```python
from build123d import *

# Parameters (mm, degrees)
ESBO_O3_R                = 2.5
RESSALTO_EXTRUS_O1_DEPTH = 7.89
ESBO_O4_W                = 8
ESBO_O4_H                = 12
RESSALTO_EXTRUS_O2_DEPTH = 10
FILETE1_R                = 10
VARREDURA1_START         = -2.055
VARREDURA1_DEPTH         = 4.5
FILETE2_R                = 10
FILETE3_R                = 1
FILETE2_OF_ESPELHAR1_R   = 10
FILETE3_OF_ESPELHAR1_R   = 1


# Read off the part's stored shape, not the designer's step: Varredura1
with BuildPart() as part:
    # Esboço3 → Ressalto-extrusão1 (new body)
    with BuildSketch(Plane.XY):
        with BuildLine():
            Line((-4, 0), (-4, 12))
            Line((-4, 12), (4, 12))
            Line((4, 12), (4, 0))
            ThreePointArc((4, 0), (0, -4), (-4, 0))
        make_face()
        Circle(ESBO_O3_R, mode=Mode.SUBTRACT)
    extrude(amount=RESSALTO_EXTRUS_O1_DEPTH)

    # Esboço4 → Ressalto-extrusão2 (add)
    with BuildSketch(Plane(origin=(0, 12, 0), x_dir=(1, 0, 0), z_dir=(0, 1, 0))):
        with Locations((0, -3.945)):
            Rectangle(ESBO_O4_W, ESBO_O4_H)
    extrude(amount=RESSALTO_EXTRUS_O2_DEPTH)

    # Filete1
    # the kernel refuses this fillet: 10 mm, written as the material it adds along each edge
    with BuildSketch(Plane(origin=(-4, 12, 0), x_dir=(0, 0, -1), z_dir=(1, 0, 0))) as filete1_piece_1:
        with BuildLine():
            CenterArc((10, -6.072641517), FILETE1_R, 142.608054869, 37.391945131)
            Line((0, -6.072641517), (-0.2, -6.072641517))
            Line((-0.2, -6.072641517), (-0.2, 0))
            Line((-0.2, 0), (0, 0.2))
            ThreePointArc((0, 0.2), (1.0275, 0.2), (1.8961, 0.12145283))
            Line((1.8961, 0.12145283), (2.055, 0))
        make_face()
    extrude(amount=8)
    with BuildSketch(Plane(origin=(-4, 12, 7.89), x_dir=(0, 0, 1), z_dir=(1, 0, 0))) as filete1_piece_2:
        with BuildLine():
            CenterArc((10, 6.072641517), FILETE1_R, 180, 37.391945131)
            Line((0, 6.072641517), (-0.2, 6.072641517))
            Line((-0.2, 6.072641517), (-0.2, 0))
            Line((-0.2, 0), (0, -0.2))
            ThreePointArc((0, -0.2), (1.0275, -0.2), (1.8961, -0.12145283))
            Line((1.8961, -0.12145283), (2.055, 0))
        make_face()
    extrude(amount=8)

    # Varredura1 outline → Varredura1 (add)
    with BuildSketch(Plane.XY.offset(VARREDURA1_START)):
        with BuildLine():
            Line((-4, 22), (4, 22))
            add(Edge.make_bspline(
                [(4, 22), (4.076004643, 24.789100523), (4.576744422, 27.046075873), (5.825537248, 29.832679333), (6.324748717, 30.661737223), (7.465829447, 32.153454516), (8.107698711, 32.816113914), (10.212438301, 34.604326425), (11.854440436, 35.53011384), (15.430236778, 37.114751087), (17.364030989, 37.773600914), (19.350774872, 38.4318674)],
                knots=[0, 0, 0, 0, 0.25, 0.25, 0.375, 0.375, 0.5, 0.5, 0.75, 0.75, 1, 1, 1, 1], degree=3))
            Line((19.350774872, 38.4318674), (16.628722538, 45.954528571))
            add(Edge.make_bspline(
                [(-4, 22), (-3.924365702, 25.610706729), (-3.278889097, 28.990240165), (-1.326924275, 33.467921051), (-0.516042652, 34.853906552), (1.338266133, 37.332612564), (2.378280036, 38.423434753), (5.639368368, 41.249638523), (7.969155498, 42.540719328), (12.436975606, 44.550100168), (14.600059443, 45.281114301), (16.628722538, 45.954528571)],
                knots=[0, 0, 0, 0, 0.25, 0.25, 0.375, 0.375, 0.5, 0.5, 0.75, 0.75, 1, 1, 1, 1], degree=3))
        make_face()
    varredura1 = extrude(amount=VARREDURA1_DEPTH)

    # Filete2
    # the kernel refuses this fillet: 10 mm, written as the material it takes off along each edge
    with BuildSketch(Plane(origin=(19.350774872, 38.4318674, -22.846513703), x_dir=(-0.9279643931477312, -0.3726688678303612, 8.125821655605385e-13), z_dir=(0, 2.1804401593599865e-12, 1.0))) as filete2_piece_1:
        with BuildLine():
            CenterArc((9.534418095, -9.925569628), FILETE2_R, 96.994915397, 71.874930906)
            Line((-0.277493979, -7.99518587), (-0.473732221, -7.956578195))
            ThreePointArc((-0.473732221, -7.956578195), (-0.338626636, -3.990655585), (-0.199879647, 0.006937349))
            Line((-0.199879647, 0.006937349), (0.012379593, 0.199616497))
            ThreePointArc((0.012379593, 0.199616497), (4.158510673, 0.013875219), (8.292249229, 0.198511393))
            Line((8.292249229, 0.198511393), (8.316605481, 0))
        make_face()
    extrude(amount=46.083027405, mode=Mode.SUBTRACT)

    # Filete3
    filete3_edges = [part.edges().sort_by_distance(p)[0] for p in [
        (16.628722538, 45.954528571, 0.195),
    ]]
    fillet(filete3_edges, radius=FILETE3_R)

    # Espelhar1: Varredura1 across plane
    add(varredura1.mirror(Plane.XY.offset(4)))

    # Filete2 of Espelhar1
    # the kernel refuses this fillet: 10 mm, written as the material it takes off along each edge
    with BuildSketch(Plane(origin=(19.350774872, 38.4318674, 30.846513703), x_dir=(-0.34025654174280723, 0.9403326463551213, 2.0503390652699583e-12), z_dir=(0, 2.1804401593599865e-12, -1.0))) as filete2_of_espelhar1_piece_1:
        with BuildLine():
            CenterArc((9.588878802, -9.87296633), FILETE2_OF_ESPELHAR1_R, 99.142350717, 71.874930906)
            Line((-0.288475994, -8.311600828), (-0.48602309, -8.280373518))
            ThreePointArc((-0.48602309, -8.280373518), (-0.158112079, -4.155526935), (-0.199925782, -0.005448096))
            Line((-0.199925782, -0.005448096), (0, 0.2))
            ThreePointArc((0, 0.2), (4, 0.2), (7.968222424, 0.197459327))
            Line((7.968222424, 0.197459327), (8, 0))
        make_face()
    extrude(amount=46.083027405, mode=Mode.SUBTRACT)

    # Filete3 of Espelhar1
    filete3_of_espelhar1_edges = [part.edges().sort_by_distance(p)[0] for p in [
        (16.628722538, 45.954528571, 7.805),
    ]]
    fillet(filete3_of_espelhar1_edges, radius=FILETE3_OF_ESPELHAR1_R)


solid = part.part
```
CAD build for the part. Positions are in the model's coordinates, mm. A direction names the side the tool comes from. Round coordinates to 2 decimals unless told otherwise and drop trailing zeros. Loops run counter-clockwise (first coordinate to the right, second up) from the corner with the lowest first, then second, coordinate; pieces in that order, holes last. Notation, with made-up numbers: M 59.25,59 L 96.25,59 A10 cw 96.25,78 Z; hole C 12.5,15 d10. An arc over 180 degrees is marked long. Return JSON: item names as keys, results as strings. Group by question number.
(1) Mould opens along Z. For faces 6 (the flat face through (6, 34, 2.445)), 7 (the flat face through (0, 22, 4)), 8 (the cylindrical face through (15.6, 39.33, 7.84)), 9 (the flat face through (0, 3, 7.89)) say: +Z half, -Z half, draft (parallel to the pull), parting line (faces both ways), or undercut.
(2) Wall check: probe 1 along Z at (x, y) = (3.25, 38) (3 decimals); probe 2 along Y at (x, z) = (0, 4.75); probe 3 along Y at (x, z) = (1.75, 1.75). Give the ranges that are in metal, low to high. Write a range as [from, to].
(3) Drop flat-ended pins along their axis: P1, Ø1.5, axis at x = 7.5, z = 3, coming from the -Y side; P2, Ø4, axis at x = 9, z = 2, coming from the +Y side; P3, Ø3.5, axis at x = 1, z = 4.5, coming from the +Y side. Give the stop position or say it passes through.
(4) Saw through at B-B, the plane z = 4.25. List the corners of the cut face in (x, y).
(5) Tool access for faces 1 (the flat face through (6, 34, 5.555)), 2 (the flat face through (0, 17, 9.945)), 3 (the flat face through (4, 11, 4)), 4 (the cylindrical face through (0, -4, 4)), 5 (the flat face through (0, 3, 0)): list every direction of +Z, -Z, +X, -X, +Y, -Y with a clear straight run to the whole face (end or side of a thin tool).
(6) Saw through at A-A, the plane y = 1.5. List the corners of the cut face in (x, z).
Answer list:
{
 "1": {"face 6": "undercut", "face 7": "undercut", "face 8": "draft", "face 9": "+Z half"},
 "2": {"probe 1": "[-2.055, 2.445], [5.555, 10.055]", "probe 2": "[-4, -2.5], [2.5, 22]", "probe 3": "[-3.6, -1.79], [1.79, 37.7]"},
 "3": {"P1": "y = 31.54", "P2": "y = 43.89", "P3": "y = 38.37"},
 "4": {"outline": "M -4,0 A4 ccw 4,0 L 4,22 L -4,22 Z; hole C 0,0 d5"},
 "5": {"face 1": "+X, -X, +Y", "face 2": "+Z, +X, -X, -Y", "face 3": "+Z, -Z, +X, -Y", "face 4": "+Z, -Z, -Y", "face 5": "-Z, +X, -X, -Y"},
 "6": {"outline": "M -4,0 L -2,0 L -2,7.89 L -4,7.89 Z; M 2,0 L 4,0 L 4,7.89 L 2,7.89 Z"}
}
